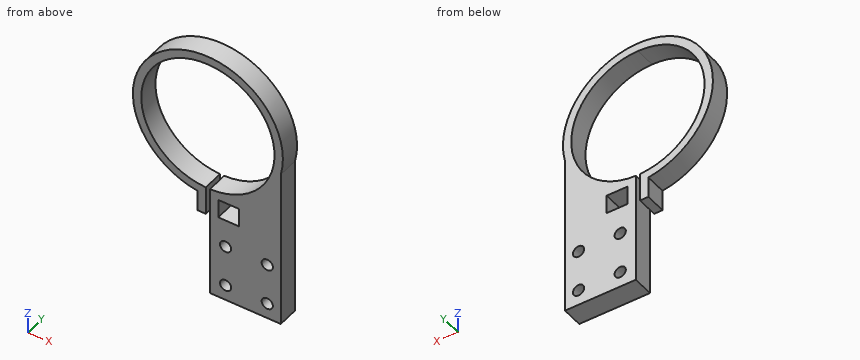
```python
from build123d import *

# Parameters (mm, degrees)
SKETCH1_R           = 45.72
SKETCH1_R_2         = 40.64
BOSS_EXTRUDE1_DEPTH = 12.7
SKETCH2_W           = 12.7
SKETCH2_H           = 12.7
BOSS_EXTRUDE2_DEPTH = 12.7
SKETCH4_W           = 2.54
SKETCH4_H           = 20.630054542
CUT_EXTRUDE2_DEPTH  = 75.919470517
BOSS_EXTRUDE3_REACH = 119.055
BOSS_EXTRUDE3_START = 38.1
SKETCH5_W           = 57.976880414
SKETCH5_H           = 12.7
SKETCH6_W           = 43.18
SKETCH6_H           = 50.8
BOSS_EXTRUDE4_DEPTH = 12.7
SKETCH7_R           = 3.429
SKETCH7_W           = 12.7
SKETCH7_H           = 11.43
CUT_EXTRUDE3_DEPTH  = 119.676105904


with BuildPart() as part:
    # Sketch1 → Boss-Extrude1 (new body)
    with BuildSketch(Plane(origin=(0, 0, 0), x_dir=(1, 0, 0), z_dir=(0, 1, 0))):
        with Locations(Location((0, 0, 0), (0, 0, 270))):
            Circle(SKETCH1_R)
        with Locations(Location((0, 0, 0), (0, 0, 270))):
            Circle(SKETCH1_R_2, mode=Mode.SUBTRACT)
    extrude(amount=BOSS_EXTRUDE1_DEPTH)

    # Sketch2 → Boss-Extrude2 (add)
    with BuildSketch(Plane(origin=(0, 0, 0), x_dir=(1, 0, 0), z_dir=(0, 1, 0))):
        with Locations((0, 51.626880414)):
            Rectangle(SKETCH2_W, SKETCH2_H)
    extrude(amount=BOSS_EXTRUDE2_DEPTH)

    # Sketch4 → Cut-Extrude2 (cut, through all)
    with BuildSketch(Plane(origin=(0, 0, 0), x_dir=(1, 0, 0), z_dir=(0, 1, 0))):
        with Locations((0, 50.104960897)):
            Rectangle(SKETCH4_W, SKETCH4_H)
    extrude(amount=CUT_EXTRUDE2_DEPTH, mode=Mode.SUBTRACT)

    # Sketch5 → Boss-Extrude3 (add, up to next)
    with BuildSketch(Plane(origin=(6.35, 0, 0), x_dir=(0, 0, -1), z_dir=(1, 0, 0)).offset(BOSS_EXTRUDE3_START), mode=Mode.PRIVATE) as boss_extrude3_sk1:
        with Locations((28.988440207, 6.35)):
            Rectangle(SKETCH5_W, SKETCH5_H)
    boss_extrude3_tool1 = extrude(boss_extrude3_sk1.sketch, amount=-BOSS_EXTRUDE3_REACH, mode=Mode.PRIVATE) - part.part
    add(boss_extrude3_tool1.solids().sort_by_distance((44.45, 6.35, -28.98844))[0])

    # Sketch6 → Boss-Extrude4 (add)
    with BuildSketch(Plane(origin=(0, 12.7, 0), x_dir=(1, 0, 0), z_dir=(0, 1, 0))):
        with Locations((22.86, 83.376880414)):
            Rectangle(SKETCH6_W, SKETCH6_H)
    extrude(amount=-BOSS_EXTRUDE4_DEPTH)

    # Sketch7 → Cut-Extrude3 (cut, through all)
    with BuildSketch(Plane(origin=(0, 0, 0), x_dir=(1, 0, 0), z_dir=(0, 1, 0))):
        with Locations(Location((10.795, 99.251880414, 0), (0, 0, 270))):
            Circle(SKETCH7_R)
        with Locations(Location((36.195, 99.251880414, 0), (0, 0, 270))):
            Circle(SKETCH7_R)
        with Locations(Location((36.195, 73.851880414, 0), (0, 0, 270))):
            Circle(SKETCH7_R)
        with Locations(Location((10.795, 73.851880414, 0), (0, 0, 270))):
            Circle(SKETCH7_R)
        with Locations((12.7, 50.991880414)):
            Rectangle(SKETCH7_W, SKETCH7_H)
    extrude(amount=CUT_EXTRUDE3_DEPTH, mode=Mode.SUBTRACT)


solid = part.part
```
Can you work these out from the model? Positions are in its coordinate system, mm. Coordinates: 2 decimals unless noted, no trailing zeros. Order: outer loops, then holes, each group sorted by start corner. A loop starts at its lowest first (then second) coordinate and runs counter-clockwise, first axis right, second up. Notation, with made-up numbers: (55.5, 71.25) - (107.5, 71.25) arc R21 cw to (107.5, 98.25) - close; hole circle Ø5 at (44.5, 36). An arc over 180 degrees is marked (long way). Answer in a Markdown table with one row per item.
1. Suppose I cut it at D-D (y = 5.5). Please give me the cut outline in (x, z) (3 decimals).
Reply:
| item | result |
|---|---|
| outline | (-6.35, -57.977) - (-1.27, -57.977) - (-1.27, -40.62) arc R40.64 cw (long way) to (1.27, -40.62) - (1.27, -108.777) - (44.45, -108.777) - (44.45, -10.701) arc R45.72 ccw (long way) to (-6.35, -45.277) - close; hole (6.35, -56.707) - (19.05, -56.707) - (19.05, -45.277) - (6.35, -45.277) - close; hole circle Ø6.858 at (10.795, -99.252); hole circle Ø6.858 at (10.795, -73.852); hole circle Ø6.858 at (36.195, -99.252); hole circle Ø6.858 at (36.195, -73.852) |
2. Suppose I cut it at C-C (z = 0). Please give me the cut outline in (x, y).
Reply:
| item | result |
|---|---|
| outline | (-45.72, 0) - (-40.64, 0) - (-40.64, 12.7) - (-45.72, 12.7) - close; (40.64, 0) - (45.72, 0) - (45.72, 12.7) - (40.64, 12.7) - close |
3. Suppose I cut it at A-A (z = -50). Please give me the cut outline in (x, y).
Reply:
| item | result |
|---|---|
| outline | (-6.35, 0) - (-1.27, 0) - (-1.27, 12.7) - (-6.35, 12.7) - close; (1.27, 0) - (6.35, 0) - (6.35, 12.7) - (1.27, 12.7) - close; (19.05, 0) - (44.45, 0) - (44.45, 12.7) - (19.05, 12.7) - close |
4. For pin 1 (5.5 mm diameter, centred on x = 10.8, z = -99.25, fed in from -Y); pin 2 (5.5 mm diameter, centred on x = -3, y = 9, fed in from -Z); pin 3 (1.5 mm diameter, centred on y = 7.5, z = -77, fed in from +X); pin 4 (6.5 mm diameter, centred on y = 9, z = -52, fed in from -X), each with a flat end and sliding along its axis, tell me the tip position at first contact or that it passes through.
Reply:
| item | result |
|---|---|
| pin 1 | passes through |
| pin 2 | stops at z = -57.98 |
| pin 3 | stops at x = 44.45 |
| pin 4 | stops at x = -6.35 |
5. If I drill on line 1 along X through (y, z) = (6.5, -46.5); line 2 along X through (y, z) = (4.5, -72); line 3 along Z through (x, y) = (36.5, 7), over which ranges is the centre line in solid material (lowest first)?
Reply:
| item | result |
|---|---|
| line 1 | x = -6.35 to -1.27, 1.27 to 6.35, 19.05 to 44.45 |
| line 2 | x = 1.27 to 7.91, 13.68 to 33.31, 39.08 to 44.45 |
| line 3 | z = -108.78 to -102.67, -95.84 to -77.27, -70.44 to -17.87, 17.87 to 27.53 |
6. Suppose I cut it at B-B (x = 25.5). Please give me the cut outline in (y, z), and give its area (3 significant figures).
Reply:
| item | result |
|---|---|
| outline | (0, -108.78) - (12.7, -108.78) - (12.7, -31.64) - (0, -31.64) - close; (0, 31.64) - (12.7, 31.64) - (12.7, 37.95) - (0, 37.95) - close |
| area | 1,060 mm^2 |
